Design review of the part built by this model. Coordinates are the model's own, in mm. A direction names the side the tool comes from. Give positions to 0.01 mm unless a question says otherwise; leave off trailing zeros. Order: outer loops, then holes, each group sorted by start corner. A loop starts at its lowest first (then second) coordinate and runs counter-clockwise, first axis right, second up. Notation, with made-up numbers: (-16, 1) - (16, 1) arc R19 cw to (16, 24) - close; hole circle Ø9 at (-2.5, 59.25). An arc over 180 degrees is marked (long way). Write each question's results on one line, items separated by ' | '. Start each with the question number.
```python
from build123d import *

# Parameters (mm, degrees)
SKETCH_1_W               = 34
SKETCH_1_H               = 41
EXTRUDE_1_DEPTH          = 5
FILLET_1_R               = 8
SKETCH_2_R               = 3.5
CUT_EXTRUDE_2_DEPTH      = 5
SKETCH_3_R               = 4
CUT_EXTRUDE_3_DEPTH      = 5
SKETCH_4_R               = 5
CUT_EXTRUDE_4_DEPTH      = 4
HOLE_WIZARD_M2_5_1_D     = 2.05
HOLE_WIZARD_M2_5_1_DEPTH = 7.35
HOLE_WIZARD_M2_5_1_TIP   = 0.615882135
CUT_EXTRUDE_5_DEPTH      = 5
SKETCH_8_R               = 1
CUT_EXTRUDE_6_DEPTH      = 5
CUT_EXTRUDE_7_DEPTH      = 2.5
SKETCH_10_R              = 3
CUT_EXTRUDE_8_DEPTH      = 1.8
SKETCH_20_W              = 5
SKETCH_20_H              = 12
EXTRUDE_1_2_DEPTH        = 3
FILLET_2_R               = 1
CUT_EXTRUDE_1_DEPTH      = 10
SKETCH_26_W              = 2
SKETCH_26_H              = 14
EXTRUDE_2_DEPTH          = 5
FILLET_3_R               = 1
FILLET_4_R               = 1
FILLET_5_R               = 1
FILLET_6_R               = 1


with BuildPart() as part:
    # 草图1 → Extrude 1 (new body)
    with BuildSketch(Plane.XY):
        with Locations((17, -20.5)):
            Rectangle(SKETCH_1_W, SKETCH_1_H)
    extrude(amount=EXTRUDE_1_DEPTH)

    # 圆角1
    fillet_1_edges = [part.edges().sort_by_distance(p)[0] for p in [
        (0, -41, 2.5),
    ]]
    fillet(fillet_1_edges, radius=FILLET_1_R)

    # 草图2 → 拉伸2 (cut)
    with BuildSketch(Plane.XY.offset(5)):
        with Locations((26, -35)):
            Circle(SKETCH_2_R)
    extrude(amount=-CUT_EXTRUDE_2_DEPTH, mode=Mode.SUBTRACT)

    # 草图3 → 拉伸3 (cut)
    with BuildSketch(Plane.XY.offset(5)):
        with Locations((5.5, -9)):
            Circle(SKETCH_3_R)
    extrude(amount=-CUT_EXTRUDE_3_DEPTH, mode=Mode.SUBTRACT)

    # 草图4 → 拉伸4 (cut)
    with BuildSketch(Plane.XY.offset(5)):
        with Locations((5.5, -9)):
            Circle(SKETCH_4_R)
    extrude(amount=-CUT_EXTRUDE_4_DEPTH, mode=Mode.SUBTRACT)

    # M2.5 螺纹孔1
    with Locations(Plane(origin=(3, 0, 2.5), x_dir=(0, 0, 1), z_dir=(0, 1, 0))):
        with Locations((0, 0), (0, 21)):
            Hole(HOLE_WIZARD_M2_5_1_D / 2, depth=HOLE_WIZARD_M2_5_1_DEPTH)
            with Locations((0, 0, -(HOLE_WIZARD_M2_5_1_DEPTH + HOLE_WIZARD_M2_5_1_TIP / 2))):  # 118° drill point
                Cone(0, HOLE_WIZARD_M2_5_1_D / 2, HOLE_WIZARD_M2_5_1_TIP, mode=Mode.SUBTRACT)

    # 草图7 → 拉伸5 (cut)
    with BuildSketch(Plane(origin=(0, 0, 0), x_dir=(-1, 0, 0), z_dir=(0, 0, -1))):
        with BuildLine():
            Line((-31.941608412, -34.164961394), (-27.140036221, 0))
            Line((-27.140036221, 0), (-34, 0))
            Line((-34, 0), (-34, -41))
            Line((-34, -41), (-26, -41))
            ThreePointArc((-26, -41), (-30.528257481, -38.936354174), (-31.941608412, -34.164961394))
        make_face()
    extrude(amount=-CUT_EXTRUDE_5_DEPTH, mode=Mode.SUBTRACT)

    # 草图8 → 拉伸6 (cut)
    with BuildSketch(Plane(origin=(0, 0, 0), x_dir=(-1, 0, 0), z_dir=(0, 0, -1))):
        with Locations((-2.5, -28)):
            Circle(SKETCH_8_R)
    extrude(amount=-CUT_EXTRUDE_6_DEPTH, mode=Mode.SUBTRACT)

    # 草图9 → 拉伸7 (cut)
    with BuildSketch(Plane(origin=(0, 0, 0), x_dir=(-1, 0, 0), z_dir=(0, 0, -1))):
        Polygon((-7.1, -31.099737486), (-0.5, -31.099737486), (-0.5, -30.7), (-0.5, -23.5), (-0.5, -22.1), (-1.9, -22.1), (-6.1, -22.1), (-7.5, -22.1), (-7.5, -23.5), (-7.5, -30.7), (-7.5, -31.099737486), align=None)
    extrude(amount=-CUT_EXTRUDE_7_DEPTH, mode=Mode.SUBTRACT)

    # 草图10 → 拉伸8 (cut)
    with BuildSketch(Plane(origin=(0, 0, 2.5), x_dir=(-1, 0, 0), z_dir=(0, 0, -1))):
        with Locations((-4, -28)):
            Circle(SKETCH_10_R)
    extrude(amount=-CUT_EXTRUDE_8_DEPTH, mode=Mode.SUBTRACT)

    # 草图20 → Extrude 1 2 (add)
    with BuildSketch(Plane.ZY):
        with Locations((2.5, -11)):
            Rectangle(SKETCH_20_W, SKETCH_20_H)
    extrude(amount=EXTRUDE_1_2_DEPTH)

    # 圆角2
    fillet_2_edges = [part.edges().sort_by_distance(p)[0] for p in [
        (0, -17, 2.5),
        (0, -5, 2.5),
        (-3, -17, 2.5),
        (-3, -5, 2.5),
    ]]
    fillet(fillet_2_edges, radius=FILLET_2_R)

    # 草图25 → 切除-拉伸1 (cut)
    with BuildSketch(Plane.XY.offset(5)):
        Polygon((0, 0), (0, -20.48158168), (-11.543504156, -18.602913064), (-5.133928875, -2.100098549), align=None)
    extrude(amount=-CUT_EXTRUDE_1_DEPTH, mode=Mode.SUBTRACT)

    # 草图26 → 凸台-拉伸2 (add)
    with BuildSketch(Plane.XY.offset(5)):
        with Locations((-1, -11)):
            Rectangle(SKETCH_26_W, SKETCH_26_H)
    extrude(amount=-EXTRUDE_2_DEPTH)

    # 圆角3
    fillet_3_edges = [part.edges().sort_by_distance(p)[0] for p in [
        (0, -4, 2.5),
    ]]
    fillet(fillet_3_edges, radius=FILLET_3_R)

    # 圆角4
    fillet_4_edges = [part.edges().sort_by_distance(p)[0] for p in [
        (0, -18, 2.5),
    ]]
    fillet(fillet_4_edges, radius=FILLET_4_R)

    # 圆角5
    fillet_5_edges = [part.edges().sort_by_distance(p)[0] for p in [
        (-2, -4, 2.5),
    ]]
    fillet(fillet_5_edges, radius=FILLET_5_R - 0.0001)  # a hair under: the kernel refuses the full size

    # 圆角6
    fillet_6_edges = [part.edges().sort_by_distance(p)[0] for p in [
        (-2, -18, 2.5),
    ]]
    fillet(fillet_6_edges, radius=FILLET_6_R - 0.0001)  # a hair under: the kernel refuses the full size


solid = part.part
```
Q1. Insertion check: pin 1 Ø2 at (x, z) = (4.5, 2) entering from -Y; pin 2 Ø3.5 at (x, y) = (3, -26.5) entering from -Z; pin 3 Ø1.5 at (y, z) = (-20, 1.5) entering from -X; pin 4 Ø1.8 at (x, y) = (2.5, -28) entering from +Z. Each pin has a flat end and moves straight along its axis. Give the tip position at first contact, or say it passes through.
Q2. Add section A-A (x = 5.5). Give the boundary of the cut face in (y, z), plus the area to 3 significant figures.
Q3. Add section B-B (y = -24). Give the boundary of the cut face in (x, z), plus the area to 3 significant figures.
Q4. For line 1 (Z direction, x = 24, y = -6) (3 decimals); line 2 (Y direction, x = 26, z = 3.65); line 3 (Y direction, x = 2.5, z = 4.6), list the stretches that pass through material, from the lowest coordinate up. Write a range as [from, to].
Q5. Draft analysis for pull direction Y (two halves, no side actions). For faces 1 (the flat face through (4, -28, 4.3)), 2 (the cylindrical face through (2, -2.16, 2.72)), 3 (the cylindrical face through (-1.715, -4.301, 2.465)), state which applies: pulls with the +Y half, pulls with the -Y half, needs draft (parallel to the pull), parting line crosses it, or undercut.
Q6. Machinability: for faces 4 (the flat face through (4, -22.1, 1)), 5 (the cylindrical face through (25.016, -3.726, 2.633)), 6 (the flat face through (-2, -11, 3)), 7 (the flat face through (0, -26, 2)), 8 (the flat face through (0, -2, 2)), which of the approach directions +Z, -Z, +X, -X, +Y, -Y give a long, thin tool a straight path to every point of the face, cutting with its end or side? Answer none if there is none.
Q7. Add section C-C (y = -18.5). Give the boundary of the cut face in (x, z).
Verdict:
1) pin 1: stops at y = -40.6 | pin 2: stops at z = 2.5 | pin 3: stops at x = 0 | pin 4: passes through
2) outline: (-40.6, 0) - (-31.1, 0) - (-31.1, 2.5) - (-30.6, 2.5) - (-30.6, 4.3) - (-25.4, 4.3) - (-25.4, 2.5) - (-22.1, 2.5) - (-22.1, 0) - (-13, 0) - (-13, 1) - (-14, 1) - (-14, 5) - (-40.6, 5) - close; (-5, 0) - (0, 0) - (0, 5) - (-4, 5) - (-4, 1) - (-5, 1) - close | area: 123 mm2
3) outline: (0, 0) - (0.5, 0) - (0.5, 2.5) - (7.5, 2.5) - (7.5, 0) - (30.51, 0) - (30.51, 5) - (0, 5) - close | area: 135 mm2
4) line 1: z = [0, 1.475], [3.525, 5] | line 2: y = [-41, -38.5], [-31.5, 0] | line 3: y = [-38.81, -29], [-27, -13], [-5, 0]
5) face 1: undercut | face 2: needs draft | face 3: pulls with the +Y half
6) face 4: -Z | face 5: +Y | face 6: +Z, -Z, -X, +Y, -Y | face 7: +Z, -Z, -X, -Y | face 8: +Z, -Z, -X, +Y
7) outline: (-0.13, 0) - (29.74, 0) - (29.74, 5) - (-0.13, 5) - close
